Geometry: final body of the model. Coordinates: model frame, mm. A direction names the side the tool comes from. Coordinates: 2 decimals unless noted, no trailing zeros. Order: outer loops, then holes, each group sorted by start corner. A loop starts at its lowest first (then second) coordinate and runs counter-clockwise, first axis right, second up. Notation, with made-up numbers: (8, -37) - (60, -37) arc R35 cw to (60, -2) - close; hole circle Ø4 at (11.5, -36.5). An arc over 180 degrees is marked (long way). Use a Markdown table: item, result. Add a question column.
```python
from build123d import *

# Parameters (mm, degrees)
BOSS_EXTRUDE1_DEPTH            = 3.175
TAP_DRILL_FOR_10_24_TAP1_D     = 3.7973
TAP_DRILL_FOR_10_24_TAP1_DEPTH = 10.16
TAP_DRILL_FOR_10_24_TAP1_TIP   = 1.140824014
CHAMFER1_SIZE                  = 2.38
CHAMFER1_EDGE_2_SIZE2          = 3.982114101
CHAMFER1_EDGE_2_SIZE           = 2.38
F_10_CLEARANCE_HOLE1_D         = 5.1054
F_10_CLEARANCE_HOLE1_DEPTH     = 12.7
F_10_CLEARANCE_HOLE1_TIP       = 1.533816902


with BuildPart() as part:
    # Sketch1 → Boss-Extrude1 (new body, symmetric)
    with BuildSketch(Plane.XY):
        Polygon((-25.4, 0), (0, 0), (13.465333043, 36.99569848), (6.304875272, 39.601891972), (-3.486612651, 12.7), (-25.4, 12.7), align=None)
    extrude(amount=BOSS_EXTRUDE1_DEPTH, both=True)

    # Tap Drill for #10-24 Tap1
    with Locations(Plane(origin=(0, 0, 0), x_dir=(-1, 0, 0), z_dir=(0, -1, 0))):
        with Locations((22.225, 0), (9.525, 0)):
            Hole(TAP_DRILL_FOR_10_24_TAP1_D / 2, depth=TAP_DRILL_FOR_10_24_TAP1_DEPTH)
            with Locations((0, 0, -(TAP_DRILL_FOR_10_24_TAP1_DEPTH + TAP_DRILL_FOR_10_24_TAP1_TIP / 2))):  # 118° drill point
                Cone(0, TAP_DRILL_FOR_10_24_TAP1_D / 2, TAP_DRILL_FOR_10_24_TAP1_TIP, mode=Mode.SUBTRACT)

    # Chamfer1
    chamfer1_edges = [part.edges().sort_by_distance(p)[0] for p in [
        (-25.4, 12.7, 0),
    ]]
    chamfer(chamfer1_edges, length=CHAMFER1_SIZE)

    # Chamfer1 edge 2
    chamfer1_edge_2_edges = [part.edges().sort_by_distance(p)[0] for p in [
        (0, 0, 0),
    ]]
    chamfer(chamfer1_edge_2_edges, length=CHAMFER1_EDGE_2_SIZE, length2=CHAMFER1_EDGE_2_SIZE2)

    # #10 Clearance Hole1
    with Locations(Plane(origin=(0, 0, 0), x_dir=(0, 0, -1), z_dir=(0.939692621, -0.342020143, 0))):
        with Locations((0, 33.02), (0, 20.32)):
            Hole(F_10_CLEARANCE_HOLE1_D / 2, depth=F_10_CLEARANCE_HOLE1_DEPTH)
            with Locations((0, 0, -(F_10_CLEARANCE_HOLE1_DEPTH + F_10_CLEARANCE_HOLE1_TIP / 2))):  # 118° drill point
                Cone(0, F_10_CLEARANCE_HOLE1_D / 2, F_10_CLEARANCE_HOLE1_TIP, mode=Mode.SUBTRACT)


solid = part.part
```
1) Draft query along X for faces 1 (the face through (1.48, 26.34, 0.04)), 2 (the face through (-7.714, 5.151, -0.57)), 3 (the face through (5.984, 16.441, 0.044)), 4 (the face through (-24.12, 5.15, -0.08)). Return one class per face: pulls with the +X half, pulls with the -X half, needs draft (parallel to the pull), parting line crosses it, or undercut.
2) Section B-B (x = -4.5). Return loops of the section in (y, z) (3 decimals), then the cut area to 3 significant figures.
3) Set-up query: faces 5 (the face through (-13, 12.7, 0)), 6 (the face through (6.889, 30.222, 1.178)). Return all of +Z, -Z, +X, -X, +Y, -Y with unobstructed straight access to the full face (end or side cutting, diameter ignored); none if empty.
4) Section C-C (z = 0.75). Give the number of separate pieces and of enclosed holes in the cut face, then the cut area to 3 significant figures.
5) Section A-A (y = 5). Return loops of the section in (x, z) (3 decimals), then the cut area to 3 significant figures.
6) Ray query, line 1 along Y through (x, z) = (-19.5, -0.25); line 2 along Z through (x, y) = (-8.5, 8) (3 decimals); line 3 along Y through (x, z) = (7, 1). Return the intervals inside material, ascending.
7) Pin query (flat end, axial travel): pin 1 (2.5 mm diameter, centred on x = -22.225, z = 0, fed in from +Y); pin 2 (1.5 mm diameter, centred on y = 24, z = 2, fed in from -X). Return the tip coordinate at first contact, or that it passes through.
Values follow:
| question | item | result |
|---|---|---|
| 1 | face 1 | pulls with the -X half |
| 1 | face 2 | undercut |
| 1 | face 3 | pulls with the +X half |
| 1 | face 4 | undercut |
| 2 | outline | (0, -3.175) - (12.7, -3.175) - (12.7, 3.175) - (0, 3.175) - close |
| 2 | area | 80.6 mm² |
| 3 | face 5 | +Z, -Z, -X, +Y |
| 3 | face 6 | none |
| 4 | separate pieces | 3 |
| 4 | enclosed holes | 0 |
| 4 | area | 404 mm² |
| 5 | outline | (-25.4, -3.175) - (1.82, -3.175) - (1.82, 3.175) - (-25.4, 3.175) - close; hole circle Ø3.797 at (-22.225, 0); hole circle Ø3.797 at (-9.525, 0) |
| 5 | area | 150 mm² |
| 6 | line 1 | y = 0 to 12.7 |
| 6 | line 2 | z = -3.175 to -1.598, 1.598 to 3.175 |
| 6 | line 3 | y = 21.58 to 30.09, 35.09 to 39.35 |
| 7 | pin 1 | stops at y = 12.7 |
| 7 | pin 2 | stops at x = 0.35 |
